from build123d import *

# Parameters (mm, degrees)
SKETCH1_R           = 6
BOSS_EXTRUDE1_DEPTH = 44.5
SHELL1_T            = -1.5
SKETCH3_R           = 3.45
BOSS_EXTRUDE3_DEPTH = 5.9
SHELL2_START        = -4.4
SHELL2_OUTLINE_R    = 1.95
SHELL2_DEPTH        = 5.9
SKETCH5_R           = 2.2
BOSS_EXTRUDE4_DEPTH = 6.4
SKETCH6_R           = 1.5
BOSS_EXTRUDE5_DEPTH = 6.4
SKETCH7_R           = 1
CUT_EXTRUDE1_DEPTH  = 12.4
SKETCH8_R           = 1.95
CUT_EXTRUDE2_DEPTH  = 51.902357509
SKETCH9_R           = 2
BOSS_EXTRUDE6_DEPTH = 11
SKETCH10_R          = 1.975
CUT_EXTRUDE3_DEPTH  = 52.730551947
SKETCH11_R          = 1
CUT_EXTRUDE4_DEPTH  = 12
BOSS_EXTRUDE8_START = -1.5
BOSS_EXTRUDE8_DEPTH = 1.5


# Read off the part's stored shape, not the designer's step: Shell2
with BuildPart() as part:
    # Sketch1 → Boss-Extrude1 (new body)
    with BuildSketch(Plane(origin=(0, 0, 0), x_dir=(1, 0, 0), z_dir=(0, 1, 0))):
        with Locations(Location((0, 0, 0), (0, 0, 270))):
            Circle(SKETCH1_R)
    extrude(amount=BOSS_EXTRUDE1_DEPTH)

    # Shell1
    shell1_openings = [part.faces().sort_by_distance(p)[0] for p in [
        (0, 44.5, 0),
    ]]
    offset(amount=SHELL1_T, openings=shell1_openings, kind=Kind.INTERSECTION)

    # Sketch3 → Boss-Extrude3 (add)
    with BuildSketch(Plane.XZ):
        with Locations(Location((0, 0, 0), (0, 0, 270))):
            Circle(SKETCH3_R)
    extrude(amount=BOSS_EXTRUDE3_DEPTH)

    # Shell2 outline → Shell2 (cut)
    with BuildSketch(Plane(origin=(0, 0, 0), x_dir=(1, 0, 0), z_dir=(0, 1, 0)).offset(SHELL2_START)):
        Circle(SHELL2_OUTLINE_R)
    extrude(amount=SHELL2_DEPTH, mode=Mode.SUBTRACT)

    # Sketch5 → Boss-Extrude4 (add)
    with BuildSketch(Plane.XY):
        with Locations(Location((0, -2.70320485, 0), (0, 0, 270))):
            Circle(SKETCH5_R)
    extrude(amount=BOSS_EXTRUDE4_DEPTH)

    # Sketch6 → Boss-Extrude5 (add)
    with BuildSketch(Plane.XY.offset(6.4)):
        with Locations((0, -2.70320485)):
            Circle(SKETCH6_R)
    extrude(amount=BOSS_EXTRUDE5_DEPTH)

    # Sketch7 → Cut-Extrude1 (cut)
    with BuildSketch(Plane.XY.offset(12.8)):
        with Locations((0, -2.70320485)):
            Circle(SKETCH7_R)
    extrude(amount=-CUT_EXTRUDE1_DEPTH, mode=Mode.SUBTRACT)

    # Sketch8 → Cut-Extrude2 (cut, through all)
    with BuildSketch(Plane(origin=(0, -4.4, 0), x_dir=(1, 0, 0), z_dir=(0, 1, 0))):
        with Locations(Location((0, 0, 0), (0, 0, 270))):
            Circle(SKETCH8_R)
    extrude(amount=CUT_EXTRUDE2_DEPTH, mode=Mode.SUBTRACT)

    # Sketch9 → Boss-Extrude6 (add)
    with BuildSketch(Plane(origin=(0, 0, 0), x_dir=(0, 0, -1), z_dir=(1, 0, 0))):
        with Locations(Location((0, -2.934503104, 0), (0, 0, 180))):
            Circle(SKETCH9_R)
    extrude(amount=BOSS_EXTRUDE6_DEPTH)

    # Sketch10 → Cut-Extrude3 (cut, through all)
    with BuildSketch(Plane(origin=(0, -4.4, 0), x_dir=(1, 0, 0), z_dir=(0, 1, 0))):
        with Locations(Location((0, -0.025, 0), (0, 0, 270))):
            Circle(SKETCH10_R)
    extrude(amount=CUT_EXTRUDE3_DEPTH, mode=Mode.SUBTRACT)

    # Sketch11 → Cut-Extrude4 (cut)
    with BuildSketch(Plane.XY.offset(12.8)):
        with Locations((0, -2.70320485)):
            Circle(SKETCH11_R)
    extrude(amount=-CUT_EXTRUDE4_DEPTH, mode=Mode.SUBTRACT)

    # Mirror5: part across plane


with BuildPart() as part_1:
    add(part.part)
    add(part.part.mirror(Plane(origin=(0, 0, 0), x_dir=(0, 0, 1), z_dir=(1, 0, 0))))

    # Sketch13 → Boss-Extrude8 (add)
    with BuildSketch(Plane(origin=(0, 44.5, 0), x_dir=(1, 0, 0), z_dir=(0, 1, 0)).offset(BOSS_EXTRUDE8_START)):
        with BuildLine():
            Line((-5.196152423, -3), (-7.95298686, -3))
            ThreePointArc((-7.95298686, -3), (-8.5, 0), (-7.95298686, 3))
            Line((-7.95298686, 3), (-5.196152423, 3))
            ThreePointArc((-5.196152423, 3), (-6, 0), (-5.196152423, -3))
        make_face()
        with BuildLine():
            Line((5.196152423, -3), (7.95298686, -3))
            ThreePointArc((7.95298686, -3), (8.5, 0), (7.95298686, 3))
            Line((7.95298686, 3), (5.196152423, 3))
            ThreePointArc((5.196152423, 3), (6, 0), (5.196152423, -3))
        make_face()
    extrude(amount=BOSS_EXTRUDE8_DEPTH)


solid = part_1.part
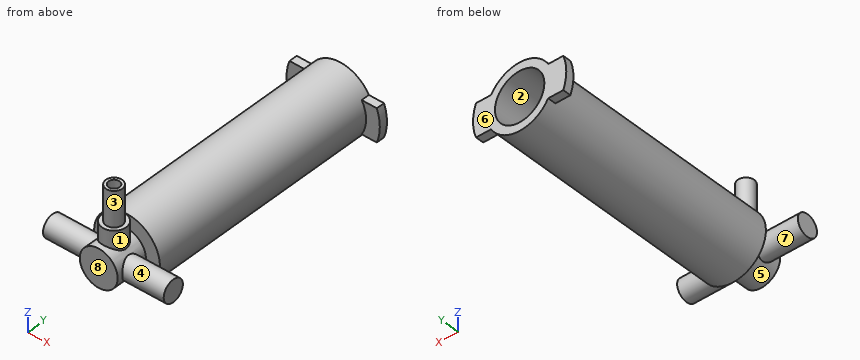
Source: CAD feature listing. Evaluate the final solid. Frame: model axes, mm. Face numbers are marked on the shaded views. A direction names the side the tool comes from. Give positions to 0.01 mm unless a question says otherwise; leave off trailing zeros. Write each loop counter-clockwise with the first axis right and the second up, starting at its lowest first coordinate (ties: lowest second). Pieces come first, ordered by that corner, then holes. Notation, with made-up numbers: M -1.75,62.5 L 3.25,62.5 A17 ccw 3.25,66.5 Z; hole C 77,6.25 d3. An arc over 180 degrees is marked long. Return JSON: item names as keys, results as strings. Group by question number.
1) Cut plane C-C, the plane z = -4. Output: boundary loops of the cut face in (x, y).
2) Set-up query: the marked faces 4, 5, 6, 7 and 8. Return all of +Z, -Z, +X, -X, +Y, -Y with unobstructed straight access to the full face (end or side cutting, diameter ignored); none if empty.
3) Material intervals for line 1 along Z through (x, y) = (0, -0.85); line 2 along Z through (x, y) = (0, -2.95); line 3 along Y through (x, z) = (-4, -3), sorted ascending. Write a range as [from, to].
4) Pull-direction query (Y, two-part tool) for the marked faces 1, 2 and 3; classes: pulls with the +Y half, pulls with the -Y half, needs draft (parallel to the pull), parting line crosses it, or undercut.
5) Cut plane A-A, the plane x = 0. Output: boundary loops of the cut face in (y, z), plus the area to 3 significant figures.
6) Cut plane D-D, the plane z = 11. Output: boundary loops of the cut face in (x, y), plus the area to 3 significant figures.
7) Cut plane B-B, the plane y = 0.5. Output: boundary loops of the cut face in (x, z) (3 decimals).
8) Pin query (flat end, axial travel): P1, Ø3.5, axis at x = 0, z = 0.025, coming from the +Y side; P2, Ø6, axis at y = 9.5, z = 3.5, coming from the -X side; P3, Ø1.6, axis at x = -6.5, y = 43.5, coming from the +Z side. Return the tip coordinate at first contact, or that it passes through.
Recorded:
{
 "1": {"outline": "M -4.47,0 L 4.47,0 L 4.47,44.5 L 2.06,44.5 L 2.06,1.5 L -2.06,1.5 L -2.06,44.5 L -4.47,44.5 Z"},
 "2": {"face 4": "+X", "face 5": "none", "face 6": "+Z, -Z, +X, -X, +Y", "face 7": "-X", "face 8": "+Z, -Z, +X, -X, -Y"},
 "3": {"line 1": "z = [-3.45, -1.95], [2, 6.4]", "line 2": "z = [-3.45, -1.95]", "line 3": "y = [0, 44.5]"},
 "4": {"face 1": "undercut", "face 2": "needs draft", "face 3": "parting line crosses it"},
 "5": {"outline": "M -5.9,-3.45 L 0,-3.45 L 0,-6 L 44.5,-6 L 44.5,-4.5 L 1.5,-4.5 L 1.5,-1.95 L -4.4,-1.95 L -4.4,2 L -3.7,2 L -3.7,12.8 L -4.2,12.8 L -4.2,6.4 L -4.9,6.4 L -4.9,3.45 L -5.9,3.45 Z; M -1.7,2 L 1.5,2 L 1.5,4.5 L 44.5,4.5 L 44.5,6 L 0,6 L 0,3.45 L -0.5,3.45 L -0.5,6.4 L -1.2,6.4 L -1.2,12.8 L -1.7,12.8 Z", "area": "175 mm²"},
 "6": {"outline": "C 0,-2.7 d3; hole C 0,-2.7 d2", "area": "3.93 mm²"},
 "7": {"outline": "C 0,0 d12; hole C 0,0.025 d3.95"},
 "8": {"P1": "stops at y = -4.4", "P2": "stops at x = -5.98", "P3": "stops at z = 3"}
}
